Verification items for the finished model (mm, model axes). Give positions to 0.01 mm unless a question says otherwise; leave off trailing zeros. Order: outer loops, then holes, each group sorted by start corner. A loop starts at its lowest first (then second) coordinate and runs counter-clockwise, first axis right, second up.
(1) Gauge pin test, flat end, axial feed: pin 1 (3 mm diameter, centred on x = 43.5, z = 74.5, fed in from +Y). Record the tip position at first contact, or that the pin passes through.
(2) Scan line: L1, parallel to Y at x = 90.5, z = 34. Record every from-to range of solid material in increasing order.
(3) Sectioned sample at B-B on z = 64. Record the cut outline in (x, y).
(4) Sectioned sample at A-A on x = 50. Record the cut outline in (y, z), plus the area to 3 significant figures.
```python
from build123d import *

# Parameters (mm, degrees)
CROQUIS1_W                    = 214
CROQUIS1_H                    = 214
SALIENTE_EXTRUIR1_DEPTH       = 2
CROQUIS2_W                    = 3
CROQUIS2_H                    = 3
SALIENTE_EXTRUIR2_DEPTH       = 0.2
CROQUIS3_W                    = 3
CROQUIS3_H                    = 3
SALIENTE_EXTRUIR3_DEPTH       = 0.2
CROQUIS4_W                    = 3
CROQUIS4_H                    = 1.5
SALIENTE_EXTRUIR4_DEPTH       = 0.2
CROQUIS5_W                    = 3
CROQUIS5_H                    = 1.5
SALIENTE_EXTRUIR5_DEPTH       = 0.2
CROQUIS6_W                    = 3
CROQUIS6_H                    = 1.5
SALIENTE_EXTRUIR6_DEPTH       = 0.2
DI_METRO_DE_TALADRO_3_0_3_1_D = 3


with BuildPart() as part:
    # Croquis1 → Saliente-Extruir1 (new body)
    with BuildSketch(Plane(origin=(0, 2, 0), x_dir=(1, 0, 0), z_dir=(0, 1, 0))):
        Rectangle(CROQUIS1_W, CROQUIS1_H)
    extrude(amount=-SALIENTE_EXTRUIR1_DEPTH)

    # Croquis2 → Saliente-Extruir2 (add)
    with BuildSketch(Plane(origin=(0, 2, 0), x_dir=(-1, 0, 0), z_dir=(0, 1, 0))):
        with Locations((-3.7, 99)):
            Rectangle(CROQUIS2_W, CROQUIS2_H)
    extrude(amount=SALIENTE_EXTRUIR2_DEPTH)

    # Croquis3 → Saliente-Extruir3 (add)
    with BuildSketch(Plane(origin=(0, 2, 0), x_dir=(-1, 0, 0), z_dir=(0, 1, 0))):
        with Locations((14.3, 99)):
            Rectangle(CROQUIS3_W, CROQUIS3_H)
    extrude(amount=SALIENTE_EXTRUIR3_DEPTH)

    # Croquis4 → Saliente-Extruir4 (add)
    with BuildSketch(Plane(origin=(0, 2, 0), x_dir=(-1, 0, 0), z_dir=(0, 1, 0))):
        with Locations((7.05, 99)):
            Rectangle(CROQUIS4_W, CROQUIS4_H)
    extrude(amount=SALIENTE_EXTRUIR4_DEPTH)

    # Croquis5 → Saliente-Extruir5 (add)
    with BuildSketch(Plane(origin=(0, 2, 0), x_dir=(-1, 0, 0), z_dir=(0, 1, 0))):
        with Locations((3.55, 97.5)):
            Rectangle(CROQUIS5_W, CROQUIS5_H)
    extrude(amount=SALIENTE_EXTRUIR5_DEPTH)

    # Croquis6 → Saliente-Extruir6 (add)
    with BuildSketch(Plane(origin=(0, 2, 0), x_dir=(-1, 0, 0), z_dir=(0, 1, 0))):
        with Locations((3.55, 100.5)):
            Rectangle(CROQUIS6_W, CROQUIS6_H)
    extrude(amount=SALIENTE_EXTRUIR6_DEPTH)

    # Diámetro de taladro Ø3.0 (3)1 (through all)
    with Locations(Plane(origin=(0, 2, 0), x_dir=(1, 0, 0), z_dir=(0, 1, 0))):
        with Locations((104.525132309, 104.525132309), (-104.525126266, -104.525126266), (104.474867691, -104.474867691), (-104.474867691, 104.474867691), (0, -104.474867691)):
            Hole(DI_METRO_DE_TALADRO_3_0_3_1_D / 2)


solid = part.part
```
Ans:
1. pin 1: stops at y = 2
2. L1: y = 0 to 2
3. outline: (-107, 0) - (107, 0) - (107, 2) - (-107, 2) - close
4. outline: (0, -107) - (2, -107) - (2, 107) - (0, 107) - close
4. area: 428 mm2
